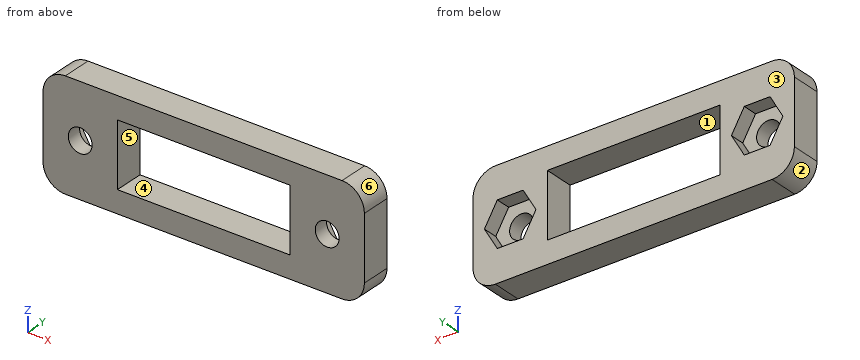
```python
from build123d import *

# Parameters (mm, degrees)
SKETCH1_W           = 43.2
SKETCH1_H           = 14.6
SKETCH1_W_2         = 23.2
SKETCH1_H_2         = 8.6
BOSS_EXTRUDE1_DEPTH = 4
CUT_EXTRUDE1_DEPTH  = 2
SKETCH5_R           = 1.6
CUT_EXTRUDE2_DEPTH  = 23.88776966
FILLET2_R           = 3


with BuildPart() as part:
    # Sketch1 → Boss-Extrude1 (new body)
    with BuildSketch(Plane(origin=(0, 0, 0), x_dir=(1, 0, 0), z_dir=(0, 1, 0))):
        Rectangle(SKETCH1_W, SKETCH1_H)
        Rectangle(SKETCH1_W_2, SKETCH1_H_2, mode=Mode.SUBTRACT)
    extrude(amount=BOSS_EXTRUDE1_DEPTH)

    # Sketch4 → Cut-Extrude1 (cut)
    with BuildSketch(Plane(origin=(0, 4, 0), x_dir=(1, 0, 0), z_dir=(0, 1, 0))):
        Polygon((18.332050808, -3), (20.064101615, 0), (18.332050808, 3), (14.867949192, 3), (13.135898385, 0), (14.867949192, -3), align=None)
        Polygon((-14.867949192, -3), (-18.332050808, -3), (-20.064101615, 0), (-18.332050808, 3), (-14.867949192, 3), (-13.135898385, 0), align=None)
    extrude(amount=-CUT_EXTRUDE1_DEPTH, mode=Mode.SUBTRACT)

    # Sketch5 → Cut-Extrude2 (cut, through all)
    with BuildSketch(Plane(origin=(0, 2, 0), x_dir=(1, 0, 0), z_dir=(0, 1, 0))):
        with Locations(Location((-16.6, 0, 0), (0, 0, 270))):
            Circle(SKETCH5_R)
        with Locations(Location((16.6, 0, 0), (0, 0, 90))):
            Circle(SKETCH5_R)
    extrude(amount=-CUT_EXTRUDE2_DEPTH, mode=Mode.SUBTRACT)

    # Fillet2
    fillet2_edges = [part.edges().sort_by_distance(p)[0] for p in [
        (-21.6, 2, -7.3),
        (21.6, 2, -7.3),
        (21.6, 2, 7.3),
        (-21.6, 2, 7.3),
    ]]
    fillet(fillet2_edges, radius=FILLET2_R)


solid = part.part
```
Can you work these out from the model? Positions are in its coordinate system, mm. Face numbers are marked on the shaded views. A direction names the side the tool comes from. Coordinates: 2 decimals unless noted, no trailing zeros. Loops run counter-clockwise (first coordinate to the right, second up) from the corner with the lowest first, then second, coordinate; pieces in that order, holes last.
1) Imagine slicing it at B-B on y = 1.6. List the corners of the cut face in (x, z) for me.
2) Imagine slicing it at C-C on z = -1. List the corners of the cut face in (x, y) for me.
3) Which directions (+Z, -Z, +X, -X, +Y, -Y) give clear straight access to the entire face, cutting with the end or side of a thin tool? Please do the marked faces 1 and 2.
4) Imagine slicing it at A-A on x = 16.6. List the corners of the cut face in (y, z) for me.
5) For pin 1 (3 mm diameter, centred on x = 16, z = 0, fed in from +Y), with a flat end and sliding along its axis, tell me the tip position at first contact or that it passes through.
6) Thinking about a two-plate mould opening in Z: for the marked faces 3, 4, 5 and 6, which applies, pulls with the +Z half, pulls with the -Z half, needs draft (parallel to the pull), parting line crosses it, or undercut?
7) I need wall thicknesses on probe 1 along X at (y, z) = (0.65, 0); probe 2 along Z at (x, y) = (16.6, 0.55); probe 3 along Z at (x, y) = (-8, 3.3). Which ranges of each line are inside material? Lowest first, please.
8) Imagine slicing it at D-D on x = -2.5. List the corners of the cut face in (y, z) for me.
Completed:
1. outline: (-21.6, -4.3) arc R3 ccw to (-18.6, -7.3) - (18.6, -7.3) arc R3 ccw to (21.6, -4.3) - (21.6, 4.3) arc R3 ccw to (18.6, 7.3) - (-18.6, 7.3) arc R3 ccw to (-21.6, 4.3) - close; hole circle Ø3.2 at (-16.6, 0); hole (-11.6, -4.3) - (11.6, -4.3) - (11.6, 4.3) - (-11.6, 4.3) - close; hole circle Ø3.2 at (16.6, 0)
2. outline: (-21.6, 0) - (-17.85, 0) - (-17.85, 2) - (-19.49, 2) - (-19.49, 4) - (-21.6, 4) - close; (-15.35, 0) - (-11.6, 0) - (-11.6, 4) - (-13.71, 4) - (-13.71, 2) - (-15.35, 2) - close; (11.6, 0) - (15.35, 0) - (15.35, 2) - (13.71, 2) - (13.71, 4) - (11.6, 4) - close; (17.85, 0) - (21.6, 0) - (21.6, 4) - (19.49, 4) - (19.49, 2) - (17.85, 2) - close
3. face 1: +Y, -Y
3. face 2: -Z, -X, +Y, -Y
4. outline: (0, -7.3) - (4, -7.3) - (4, -3) - (2, -3) - (2, -1.6) - (0, -1.6) - close; (0, 1.6) - (2, 1.6) - (2, 3) - (4, 3) - (4, 7.3) - (0, 7.3) - close
5. pin 1: stops at y = 2
6. face 3: needs draft
6. face 4: undercut
6. face 5: undercut
6. face 6: pulls with the +Z half
7. probe 1: x = -21.6 to -18.2, -15 to -11.6, 11.6 to 15, 18.2 to 21.6
7. probe 2: z = -7.3 to -1.6, 1.6 to 7.3
7. probe 3: z = -7.3 to -4.3, 4.3 to 7.3
8. outline: (0, -7.3) - (4, -7.3) - (4, -4.3) - (0, -4.3) - close; (0, 4.3) - (4, 4.3) - (4, 7.3) - (0, 7.3) - close
